Design review of the part built by this model. Coordinates are the model's own, in mm. Face numbers are marked on the shaded views. A direction names the side the tool comes from. Coordinates: 2 decimals unless noted, no trailing zeros. Write each loop counter-clockwise with the first axis right and the second up, starting at its lowest first coordinate (ties: lowest second). Pieces come first, ordered by that corner, then holes. Notation, with made-up numbers: (-35.5, 29) - (11.5, 29) arc R10 cw to (11.5, 43) - close; hole circle Ø11 at (89.5, -31). An arc over 180 degrees is marked (long way). Answer as a JSON object with one key per item and string values.
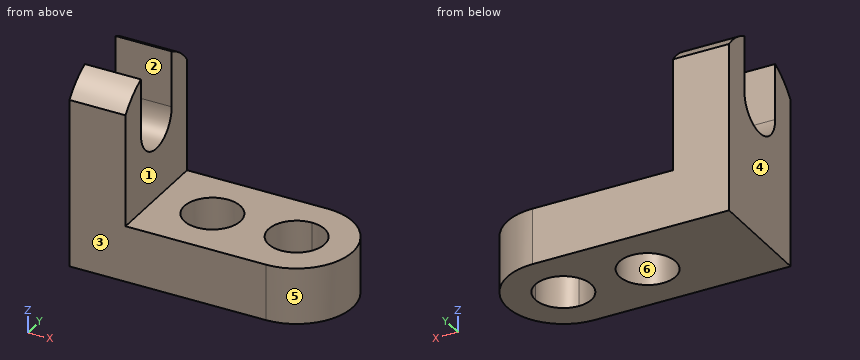
```python
from build123d import *

# Parameters (mm, degrees)
F1_DEPTH = 25.4
F2_W     = 12.7
F2_H     = 7.675322
F3_DEPTH = 12.7
F4_DEPTH = 12.7
F5_R     = 6.35
F6_DEPTH = 25.4
F7_DEPTH = 12.7


with BuildPart() as f1:
    # F0 (on Front) → F1 (new body)
    with BuildSketch(Plane.XZ):
        Polygon((0, 38.1), (0, 0), (44.45, 0), (44.45, 12.7), (12.7, 12.7), (12.7, 38.1), align=None)
    extrude(amount=F1_DEPTH)

    # F2 (on face) → F3 (cut)
    with BuildSketch(Plane(origin=(0, 0, 0), x_dir=(0, -1, 0), z_dir=(-1, 0, 0))):
        with BuildLine():
            Line((6.35, 38.1), (6.35, 43.124678))
            ThreePointArc((6.35, 43.124678), (2.84924, 41.024022), (0, 38.1))
            Line((0, 38.1), (6.35, 38.1))
        make_face()
        with Locations((12.7, 34.262339)):
            Rectangle(F2_W, F2_H)
        with BuildLine():
            ThreePointArc((6.35, 30.424678), (12.7, 24.074678), (19.05, 30.424678))
            Line((19.05, 30.424678), (6.35, 30.424678))
        make_face()
    extrude(amount=-F3_DEPTH, mode=Mode.SUBTRACT)

    # F2 (on face) → F4 (join)
    with BuildSketch(Plane(origin=(0, 0, 0), x_dir=(0, -1, 0), z_dir=(-1, 0, 0))):
        with BuildLine():
            Line((6.35, 38.1), (6.35, 43.124678))
            ThreePointArc((6.35, 43.124678), (2.84924, 41.024022), (0, 38.1))
            Line((0, 38.1), (6.35, 38.1))
        make_face()
        with BuildLine():
            Line((19.05, 38.1), (25.4, 38.1))
            ThreePointArc((25.4, 38.1), (22.55076, 41.024022), (19.05, 43.124678))
            Line((19.05, 43.124678), (19.05, 38.1))
        make_face()
    extrude(amount=-F4_DEPTH)

    # F5 (on face) → F6 (cut)
    with BuildSketch(Plane.XY.offset(12.7)):
        with BuildLine():
            Line((44.45, -6.35), (44.45, -19.05))
            ThreePointArc((44.45, -19.05), (48.940128, -17.190128), (50.8, -12.7))
            ThreePointArc((50.8, -12.7), (48.940128, -8.209872), (44.45, -6.35))
        make_face()
        with BuildLine():
            ThreePointArc((44.45, -6.35), (38.1, -12.7), (44.45, -19.05))
            Line((44.45, -19.05), (44.45, -6.35))
        make_face()
        with Locations((25.4, -12.7)):
            Circle(F5_R)
    extrude(amount=-F6_DEPTH, mode=Mode.SUBTRACT)

    # F5 (on face) → F7 (join)
    with BuildSketch(Plane.XY.offset(12.7)):
        with BuildLine():
            Line((44.45, -19.05), (44.45, -25.4))
            ThreePointArc((44.45, -25.4), (57.15, -12.7), (44.45, 0))
            Line((44.45, 0), (44.45, -6.35))
            ThreePointArc((44.45, -6.35), (48.940128, -8.209872), (50.8, -12.7))
            ThreePointArc((50.8, -12.7), (48.940128, -17.190128), (44.45, -19.05))
        make_face()
    extrude(amount=-F7_DEPTH)


solid = f1.part
```
(1) Take a section at A-A, the plane z = 5.5. Write out the cut boundary in (x, y).
Solved:
{"outline": "(0, -25.4) - (44.45, -25.4) arc R12.7 ccw to (44.45, 0) - (0, 0) - close; hole circle Ø12.7 at (25.4, -12.7); hole circle Ø12.7 at (44.45, -12.7)"}
(2) Take a section at C-C, the plane y = -16.75. Write out the cut boundary in (x, z).
Solved:
{"outline": "(0, 0) - (20.51, 0) - (20.51, 12.7) - (12.7, 12.7) - (12.7, 25.53) - (0, 25.53) - close; (30.29, 0) - (39.56, 0) - (39.56, 12.7) - (30.29, 12.7) - close; (49.34, 0) - (56.49, 0) - (56.49, 12.7) - (49.34, 12.7) - close"}
(3) To check wall thickness, follow line 1 (X direction, y = -11, z = 12.5); line 2 (Y direction, x = 25.4, z = 6); line 3 (Z direction, x = 25, y = -4.25). State the ranges of each line that lie inside material, in increasing order. Write a range as from..to.
Solved:
{"line 1": "x = 0..19.28, 31.52..38.33, 50.57..57.04", "line 2": "y = -25.4..-19.05, -6.35..0", "line 3": "z = 0..12.7"}
(4) For pin 1 (3 mm diameter, centred on y = -22.5, z = 32.5, fed in from +X); pin 2 (3 mm diameter, centred on x = 27, y = -7.5, fed in from +Z), all flat-tipped, find the tip position at first contact; note any pin that passes through.
Solved:
{"pin 1": "stops at x = 12.7", "pin 2": "stops at z = 12.7"}
(5) The part is to be moulded in two halves that separate along X. For the marked faces 4, 5 and 6, say which applies: pulls with the +X half, pulls with the -X half, needs draft (parallel to the pull), parting line crosses it, or undercut.
Solved:
{"face 4": "pulls with the -X half", "face 5": "pulls with the +X half", "face 6": "undercut"}
(6) Take a section at D-D, the plane z = 26.5. Write out the cut boundary in (x, y).
Solved:
{"outline": "(0, -25.4) - (12.7, -25.4) - (12.7, -17.69) - (0, -17.69) - close; (0, -7.71) - (12.7, -7.71) - (12.7, 0) - (0, 0) - close"}
(7) Take a section at B-B, the plane x = 25.4. Write out the cut boundary in (y, z), and give its area (3 significant figures).
Solved:
{"outline": "(-25.4, 0) - (-19.05, 0) - (-19.05, 12.7) - (-25.4, 12.7) - close; (-6.35, 0) - (0, 0) - (0, 12.7) - (-6.35, 12.7) - close", "area": "161 mm^2"}
(8) Tool access review of the marked faces 1, 2 and 3: name each direction out of +Z, -Z, +X, -X, +Y, -Y from which nothing blocks a thin tool from reaching the whole face with its end or side.
Solved:
{"face 1": "+Z, +X, +Y, -Y", "face 2": "+Z, +X, -X", "face 3": "+Z, -Z, +X, -X, -Y"}
